Autodesk Inventor part; units mm, degrees
ref_plane "YZ Plane" through (0, 0, 0) normal (1, 0, 0) x (0, 1, 0)
ref_plane "XZ Plane" through (0, 0, 0) normal (0, 1, 0) x (-1, 0, 0)
ref_plane "XY Plane" through (0, 0, 0) normal (0, 0, 1) x (1, 0, 0)
sketch "Sketch1" plane through (0, 0, 0) normal (0, 1, 0) x (-1, 0, 0)
  line L0 (-7.5, 5.5) -> (7.5, 5.5)
  line L1 (7.5, 5.5) -> (7.5, -5.5)
  line L2 (7.5, -5.5) -> (-7.5, -5.5)
  line L3 (-7.5, -5.5) -> (-7.5, 5.5)
  line L4 (-7.5, 5.5) -> (7.5, -5.5) construction
  line L5 (7.5, 5.5) -> (-7.5, -5.5) construction
  circle A0 centre (0, -5.5) radius 7.5 construction
  arc A1 (-7.5, -5.5) -> (7.5, -5.5) centre (0, -5.5) ccw
  point P0 (0, 0)
  dimension "d0" = 11
  dimension "d1" = 15
extrude "Extrusion1" add sketch "Sketch1" along normal blind 8
sketch "Sketch2" plane through (0, 0, 0) normal (0, -1, 0) x (1, 0, 0)
  line L0 (7.5, 9.25) -> (-7.5, 9.25)
  line L1 (-7.5, 9.25) -> (-7.5, -20.75)
  line L2 (-7.5, -20.75) -> (7.5, -20.75)
  line L3 (7.5, -20.75) -> (7.5, 9.25)
  line L4 (7.5, 9.25) -> (-7.5, -20.75) construction
  line L5 (-7.5, 9.25) -> (7.5, -20.75) construction
  line L6 (-7.5, 5.5) -> (7.5, 5.5)
  line L7 (7, 8.75) -> (-7, 8.75) construction
  line L8 (-7, 8.75) -> (-7, -20.25) construction
  line L9 (-7, -20.25) -> (7, -20.25) construction
  line L10 (7, -20.25) -> (7, 8.75) construction
  line L11 (7, 8.75) -> (-7, -20.25) construction
  line L12 (-7, 8.75) -> (7, -20.25) construction
  point P0 (0, 0)
  point P1 (0, -5.75)
  dimension "d4" = 15
  dimension "d5" = 30
  dimension "d6" = 3.75
  dimension "d18" = 0.5
  dimension "d19" = 0.5
sketch "Sketch4" plane through (0, 0, 0) normal (0, -1, 0) x (1, 0, 0)
  line L0 (-7.5, -5.5) -> (-7.5, 5.5)
  line L1 (-7.5, 3.75) -> (-6.5, 3.75)
  line L2 (-6.5, 3.75) -> (-6.5, 0.75)
  line L3 (-6.5, 0.75) -> (-7.5, 0.75)
  line L4 (-7.5, 0.75) -> (-7.5, 3.75)
  line L5 (7.5, 5.5) -> (7.5, -5.5)
  line L6 (7.5, 0.75) -> (6.5, 0.75)
  line L7 (6.5, 0.75) -> (6.5, 3.75)
  line L8 (6.5, 3.75) -> (7.5, 3.75)
  line L9 (7.5, 3.75) -> (7.5, 0.75)
  line L10 (-7.5, -20.25) -> (7.5, -20.25) construction
  line L11 (7.5, -20.25) -> (7.5, 9.75) construction
  line L12 (7.5, 9.75) -> (-7.5, 9.75) construction
  line L13 (-7.5, 9.75) -> (-7.5, -20.25) construction
  line L14 (-7.5, -20.25) -> (7.5, 9.75) construction
  line L15 (7.5, -20.25) -> (-7.5, 9.75) construction
  line L16 (-7.5, 5.5) -> (7.5, 5.5) construction
  arc A0 (-7.5, -5.5) -> (7.5, -5.5) centre (0, -5.5) ccw construction
  point P0 (0, 0)
  point P1 (0, -5.25)
  point P2 (0, -13)
  point P3 (-7, 3.75)
  point P4 (-7.5, 0.75)
  point P5 (-7, 0.75)
  point P6 (7.5, 3.75)
  point P7 (-7.5, 0.75)
  dimension "d20" = 1
  dimension "d21" = 3
  dimension "d22" = 1
  dimension "d23" = 3
  dimension "d24" = 15
  dimension "d25" = 30
  dimension "d27" = 7.25
  dimension "d106" = 0.75
extrude "Extrusion3" add sketch "Sketch4" along normal blind 1.6
sketch "Sketch6" plane through (0, 0, 0) normal (0, -1, 0) x (1, 0, 0)
  line L0 (7.5, 11.25) -> (-7.5, 11.25)
  line L1 (-7.5, 11.25) -> (-7.5, -18.75)
  line L2 (-7.5, -18.75) -> (7.5, -18.75)
  line L3 (7.5, -18.75) -> (7.5, 11.25)
  line L4 (7.5, 11.25) -> (-7.5, -18.75) construction
  line L5 (-7.5, 11.25) -> (7.5, -18.75) construction
  line L6 (7, 10.75) -> (-7, 10.75) construction
  line L7 (-7, 10.75) -> (-7, -18.25) construction
  line L8 (-7, -18.25) -> (7, -18.25) construction
  line L9 (7, -18.25) -> (7, 10.75) construction
  line L10 (7, 10.75) -> (-7, -18.25) construction
  line L11 (-7, 10.75) -> (7, -18.25) construction
  circle A0 centre (0, -3.75) radius 1
  circle A1 centre (0, -3.75) radius 1.5
  line L12 (-6.5, 4.5) -> (6.5, 4.5)
  line L13 (6.5, 4.5) -> (6.5, -5.5)
  line L14 (6.5, -5.5) -> (-6.5, -5.5)
  line L15 (-6.5, -5.5) -> (-6.5, 4.5)
  line L16 (-7.5, 5.5) -> (7.5, 5.5)
  arc A2 (-7.5, -5.5) -> (7.5, -5.5) centre (0, -5.5) ccw
  circle A3 centre (0, -5.5) radius 6.5
  point P0 (0, 0)
  point P1 (-7.5, -3.75)
  point P2 (6.5, -5.5)
  dimension "d31" = 15
  dimension "d32" = 30
  dimension "d34" = 0.5
  dimension "d35" = 0.5
  dimension "d36" = 2
  dimension "d37" = 0.5
  dimension "d38" = 1
  dimension "d39" = 1
  dimension "d40" = 1
  dimension "d41" = 1
  dimension "d107" = 3.75
extrude "Extrusion4" cut sketch "Sketch6" against normal blind 2.5 contours A0 | L12 L13 A3 L15 | A3 L14 | L14 A3
sketch "Sketch10" plane through (0, 8, 0) normal (0, 1, 0) x (1, 0, 0)
  point P0 (0, 0)
sketch "Sketch11" plane through (0, 0, 0) normal (0, -1, 0) x (1, 0, 0)
  line L0 (-5, 3.5) -> (-2.5, 3.5)
  line L1 (-2.5, 3.5) -> (-2.5, 2)
  line L2 (-2.5, 2) -> (-5, 2)
  line L3 (-5, 2) -> (-5, 3.5)
  line L4 (2.5, 3.5) -> (5, 3.5)
  line L5 (5, 3.5) -> (5, 2)
  line L6 (5, 2) -> (2.5, 2)
  line L7 (2.5, 2) -> (2.5, 3.5)
  line L8 (-6.5, 3.75) -> (-7.5, 3.75)
  line L9 (-6.5, 0.75) -> (-6.5, 3.75)
  line L10 (6.5, 3.75) -> (6.5, 0.75)
  line L11 (-6.5, 4.5) -> (6.5, 4.5)
  line L12 (-1.25, -11) -> (1.25, -11)
  line L13 (1.25, -11) -> (1.25, -9.5)
  line L14 (1.25, -9.5) -> (-1.25, -9.5)
  line L15 (-1.25, -9.5) -> (-1.25, -11)
  circle A0 centre (0, -3.75) radius 1
  point P0 (0, 0)
  point P1 (-3.75, 3.5)
  point P2 (3.75, 3.5)
  point P3 (1.25, -10.25)
  point P4 (2.5, 2.75)
  point P5 (0, -9.5)
  point P6 (3.75, 2)
  point P7 (-2.5, 2.75)
  dimension "d51" = 2.5
  dimension "d52" = 1.5
  dimension "d55" = 2.75
  dimension "d56" = 2.75
  dimension "d60" = 13
  dimension "d61" = 3.75
  dimension "d62" = 3.75
  dimension "d103" = 6.5
  dimension "d104" = 6.5
extrude "Extrusion8" cut sketch "Sketch11" against normal blind 10 contours L0 L1 L2 L3 | L4 L5 L6 L7 | L15 L14 L13 L12
sketch "Sketch12" plane through (0, 2.5, 0) normal (0, -1, 0) x (1, 0, 0)
  line L0 (5, 2) -> (5, 3.5) construction
  line L1 (2.5, 2) -> (5, 2) construction
  line L2 (5, 3.5) -> (2.5, 3.5) construction
  line L3 (2.5, 3.5) -> (2.5, 2) construction
  line L4 (2.5, 2) -> (5, 2) construction
  line L5 (5, 2) -> (5, 3.5) construction
  line L6 (-2.5, 2) -> (-2.5, 3.5) construction
  line L7 (-2.5, 2) -> (-5, 2) construction
  line L8 (-2.5, 3.5) -> (-5, 3.5) construction
  line L9 (-5, 3.5) -> (-5, 2) construction
  line L10 (-5, 2) -> (-2.5, 2) construction
  line L11 (-2.5, 2) -> (-2.5, 3.5) construction
  line L12 (-1.25, -9.5) -> (1.25, -9.5) construction
  line L13 (-1.25, -9.5) -> (-1.25, -11) construction
  line L14 (1.25, -9.5) -> (-1.25, -9.5) construction
  line L15 (-1.25, -9.5) -> (-1.25, -11) construction
  line L16 (-1.25, -11) -> (1.25, -11) construction
  line L17 (1.25, -11) -> (1.25, -9.5) construction
  line L18 (5.5, 3.5) -> (2, 3.5)
  line L19 (2, 3.5) -> (2, 2)
  line L20 (2, 2) -> (5.5, 2)
  line L21 (5.5, 2) -> (5.5, 3.5)
  line L22 (1.75, -9.5) -> (-1.75, -9.5)
  line L23 (-1.75, -9.5) -> (-1.75, -11)
  line L24 (-1.75, -11) -> (1.75, -11)
  line L25 (1.75, -11) -> (1.75, -9.5)
  line L26 (-2, 3.5) -> (-5.5, 3.5)
  line L27 (-5.5, 3.5) -> (-5.5, 2)
  line L28 (-5.5, 2) -> (-2, 2)
  line L29 (-2, 2) -> (-2, 3.5)
  point P0 (0, 0)
  point P1 (-2.5, 2.75)
  point P2 (-2, 2.75)
  point P3 (-3.75, 2)
  point P4 (-3.75, 2)
  point P5 (-3.75, 3.5)
  point P6 (-3.75, 3.5)
  point P7 (-5, 2.75)
  point P8 (-5.5, 2.75)
  point P9 (1.25, -10.25)
  point P10 (1.75, -10.25)
  point P11 (0, -11)
  point P12 (-1.25, -10.25)
  dimension "d63" = 0.5
  dimension "d64" = 0
  dimension "d65" = 0
  dimension "d67" = 0.5
  dimension "d68" = 0
  dimension "d69" = 0
  dimension "d70" = 0.5
  dimension "d71" = 0.5
  dimension "d72" = 0
  dimension "d73" = 0
  dimension "d74" = 0.5
  dimension "d96" = 0.5
extrude "Extrusion9" cut sketch "Sketch12" against normal blind 1
sketch "Sketch16" plane through (0, 2.5, 0) normal (0, -1, 0) x (1, 0, 0)
  line L0 (-6.5, -5.5) -> (-6.5, 4.5) construction
  line L1 (-6.5, 4.5) -> (6.5, 4.5) construction
  line L2 (-6.5, 4.5) -> (6.5, 4.5) construction
  line L3 (-0.5, 4.5) -> (0.5, 4.5)
  line L4 (0.5, 4.5) -> (0.5, -2.75)
  line L5 (0.5, -2.75) -> (-0.5, -2.75)
  line L6 (-0.5, -2.75) -> (-0.5, 4.5)
  circle A0 centre (0, -3.75) radius 1.5 construction
  circle A1 centre (0, -3.75) radius 1.75 construction
  line L7 (-6.5, -2.75) -> (6.5174, -2.75) construction
  circle A2 centre (0, -3.75) radius 1.5 construction
  circle A3 centre (0, -3.75) radius 1 construction
  line L8 (6.5, 0.75) -> (6.5, -5.5)
  line L9 (-6.5, -5.873) -> (6.5, -5.873)
  line L10 (6.5, -5.873) -> (6.5, -6.873)
  line L11 (6.5, -6.873) -> (-6.5, -6.873)
  line L12 (-6.5, -6.873) -> (-6.5, -5.873)
  point P0 (0, 0)
  point P1 (0, 4.5)
  point P2 (0.0087, -2.75)
  dimension "d94" = 1
  dimension "d95" = 1
extrude "Extrusion10" add sketch "Sketch16" along normal blind 2.5 contours L3 L4 L5 L6
sketch "Sketch18" plane through (0, 2.5, -3.75) normal (0, -1, 0) x (1, 0, 0)
  circle A0 centre (0, 0) radius 1
  circle A1 centre (0, 0) radius 1
  point P0 (0, 3.75)
extrude "Extrusion12" cut sketch "Sketch18" against normal blind 3
sketch "Sketch14" plane through (0, 2.5, 0) normal (0, -1, 0) x (1, 0, 0)
  line L0 (5, 2.75) -> (2.5, 2.75) construction
  line L1 (2.5, 2.75) -> (2.5, 1.25) construction
  line L2 (2.5, 1.25) -> (5, 1.25) construction
  line L3 (5, 1.25) -> (5, 2.75) construction
  line L4 (5.5, 3.25) -> (2, 3.25)
  line L5 (2, 3.25) -> (2, 0.75)
  line L6 (2, 0.75) -> (5.5, 0.75)
  line L7 (5.5, 0.75) -> (5.5, 3.25)
  dimension "d86" = 0.5
  dimension "d87" = 0.5
sketch "Sketch15" plane through (0, 3.5, 0) normal (0, -1, 0) x (1, 0, 0)
  line L0 (5, 2.75) -> (2.5, 2.75)
  line L1 (2.5, 2.75) -> (2.5, 1.25)
  line L2 (2.5, 1.25) -> (5, 1.25)
  line L3 (5, 1.25) -> (5, 2.75)
  point P0 (0, 0)
sketch "Sketch8" plane through (0, 0, -3.75) normal (0, -1, 0) x (1, 0, 0)
  circle A0 centre (0, 0) radius 1.75
  circle A1 centre (0, 0) radius 1.5
  circle A2 centre (0, 0) radius 1.5
  point P0 (0, 3.75)
  dimension "d46" = 0.25
sketch "Sketch7" plane through (0, 2.5, -3.75) normal (0, -1, 0) x (1, 0, 0)
  circle A0 centre (0, 0) radius 1.25
  point P0 (0, 3.75)
properties part number "ANDGATE"
Work out the finished part from the listing and answer in its coordinate system (mm). A direction names the side the tool comes from. Round coordinates to 2 decimals unless told otherwise and drop trailing zeros. Write each loop counter-clockwise with the first axis right and the second up, starting at its lowest first coordinate (ties: lowest second). Pieces come first, ordered by that corner, then holes. Notation, with made-up numbers: M 59,6 L 113,6 A12 ccw 113,16 Z; hole C 86.5,86 d9. An arc over 180 degrees is marked long. Use a Markdown table: item, result.
1) The part is cut by section D-D on y = 2. Give the vertices of the cut face in (x, z), plus the area to 3 significant figures.
Taken from the geometry:
| item | result |
|---|---|
| outline | M -7.5,-5.5 A7.5 ccw 7.5,-5.5 L 7.5,5.5 L -7.5,5.5 Z; hole M -6.5,-5.5 A6.5 ccw 6.5,-5.5 L 6.5,4.5 L 0.5,4.5 L 0.5,-2.34 A1.5 cw long -0.5,-2.34 L -0.5,4.5 L -6.5,4.5 Z; hole C 0,-3.75 d2 |
| area | 67.7 mm2 |
2) The part is cut by section C-C on z = 0. Give the vertices of the cut face in (x, y), plus the area to 3 significant figures.
Taken from the geometry:
| item | result |
|---|---|
| outline | M -7.5,0 L -6.5,0 L -6.5,2.5 L -0.5,2.5 L -0.5,0 L 0.5,0 L 0.5,2.5 L 6.5,2.5 L 6.5,0 L 7.5,0 L 7.5,8 L -7.5,8 Z |
| area | 90.0 mm2 |
3) Consider line 1 (Z direction, x = 0, y = 4.45); line 2 (Z direction, x = 0, y = 1.3); line 3 (X direction, y = 2, z = -5.5). Determine where each line is inside the solid, lowest interval first. Write a range as [from, to].
Taken from the geometry:
| item | result |
|---|---|
| line 1 | z = [-13, -11], [-9.5, -4.75], [-2.75, 5.5] |
| line 2 | z = [-13, -12], [-5.25, -4.75], [-2.75, 5.5] |
| line 3 | x = [-7.5, -6.5], [6.5, 7.5] |
4) The part is cut by section B-B on x = 0. Give the vertices of the cut face in (y, z), plus the area to 3 significant figures.
Taken from the geometry:
| item | result |
|---|---|
| outline | M 0,-13 L 8,-13 L 8,-11 L 2.5,-11 L 2.5,-12 L 0,-12 Z; M 0,-5.25 L 2.5,-5.25 L 2.5,-9.5 L 8,-9.5 L 8,5.5 L 0,5.5 L 0,-2.75 L 5.5,-2.75 L 5.5,-4.75 L 0,-4.75 Z |
| area | 112 mm2 |
5) Flat-ended cylindrical pins translate along their axes: pin 1 (0.8 mm diameter, centred on x = -7, y = -0.5, fed in from +Z); pin 2 (3 mm diameter, centred on y = 5.5, z = -7.5, fed in from +X); pin 3 (0.6 mm diameter, centred on x = -2, z = 2.5, fed in from -Y). Find the tip coordinate at first contact, or state that the pin passes through.
Taken from the geometry:
| item | result |
|---|---|
| pin 1 | stops at z = 3.75 |
| pin 2 | stops at x = 7.48 |
| pin 3 | stops at y = 2.5 |
6) Which of the six approach directions +Z, -Z, +X, -X, +Y, -Y give full straight-line access (tool end or side, diameter ignored) to faces 4 (the face through (7, -1, 0.75)), 5 (the face through (-2, 3, 3)), 6 (the face through (-2.5, 6, 3))?
Taken from the geometry:
| item | result |
|---|---|
| face 4 | -Z, +X, -X, -Y |
| face 5 | -Y |
| face 6 | +Y, -Y |
7) Determine the mould class of faces 1 (the face through (0, 4, -13)), 2 (the face through (4, 5, 3.5)), 3 (the face through (7, -1, 3.75)) for opening direction X: pulls with the +X half, pulls with the -X half, needs draft (parallel to the pull), parting line crosses it, or undercut.
Taken from the geometry:
| item | result |
|---|---|
| face 1 | parting line crosses it |
| face 2 | undercut |
| face 3 | needs draft |
8) The part is cut by section A-A on y = 6.75. Give the vertices of the cut face in (x, z).
Taken from the geometry:
| item | result |
|---|---|
| outline | M -7.5,-5.5 A7.5 ccw 7.5,-5.5 L 7.5,5.5 L -7.5,5.5 Z; hole M -5,2 L -2.5,2 L -2.5,3.5 L -5,3.5 Z; hole M -1.25,-11 L 1.25,-11 L 1.25,-9.5 L -1.25,-9.5 Z; hole M 2.5,2 L 5,2 L 5,3.5 L 2.5,3.5 Z |
